Can you work these out from the model? Positions are in its coordinate system, mm. Give positions to 0.01 mm unless a question says otherwise; leave off trailing zeros. Loops run counter-clockwise (first coordinate to the right, second up) from the corner with the lowest first, then second, coordinate; pieces in that order, holes last. Notation, with made-up numbers: (75, -8.75) -> (124, -8.75) arc R25 ccw to (124, 28.25) -> close; hole circle Ø3 at (-16.75, 86.25). An arc over 180 degrees is marked (long way). One line per question, with ' | ' between items.
from build123d import *

# Parameters (mm, degrees)
F0_W     = 589.788
F0_H     = 50.8
F1_DEPTH = 50.8
F2_DEPTH = 50.8
F3_DEPTH = 50.8


with BuildPart() as f1:
    # F0 (on Front) → F1 (new body)
    with BuildSketch(Plane.XZ):
        with Locations((294.894, 25.4)):
            Rectangle(F0_W, F0_H)
    extrude(amount=F1_DEPTH)

    # F0 (on Front) → F2 (join)
    with BuildSketch(Plane.XZ):
        Polygon((589.788, 50.8), (589.788, 0), (596.061459, 0), align=None)
    extrude(amount=F2_DEPTH)

    # F0 (on Front) → F3 (join)
    with BuildSketch(Plane.XZ):
        Polygon((-6.273459, 0), (0, 0), (0, 50.8), align=None)
    extrude(amount=F3_DEPTH)


solid = f1.part
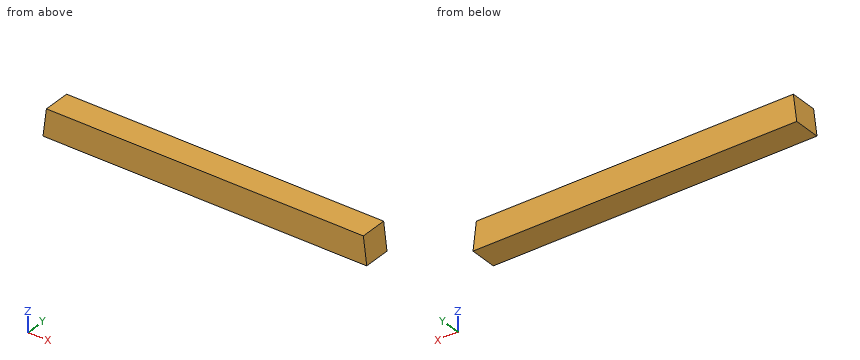
Q1. For pin 1 Ø1 at (y, z) = (-11, 31.5) entering from -X; pin 2 Ø10 at (y, z) = (-14.5, 44) entering from +X; pin 3 Ø6 at (y, z) = (-35.5, 20) entering from -X, each with a flat end and sliding along its axis, tell me the tip position at first contact or that it passes through.
Entries:
pin 1: x = -2.45 | pin 2: x = 591.25 | pin 3: x = -4.17
Q2. If I drill on probe 1 along X at (y, z) = (-6, 31); probe 2 along X at (y, z) = (-30.5, 35), over which ranges is the centre line in solid material (lowest first)? Write a range as from..to.
Entries:
probe 1: -2.45..592.23 | probe 2: -1.95..591.74
Q3. If we section it at A-A (z = 39): Write out the boundary of the cut face in (x, y).
Entries:
outline: (-1.46, -50.8) -> (591.25, -50.8) -> (591.25, 0) -> (-1.46, 0) -> close
